Autodesk Inventor part; units mm, degrees
ref_plane "YZ Plane" through (0, 0, 0) normal (1, 0, 0) x (0, 1, 0)
ref_plane "XZ Plane" through (0, 0, 0) normal (0, 1, 0) x (-1, 0, 0)
ref_plane "XY Plane" through (0, 0, 0) normal (0, 0, 1) x (1, 0, 0)
sketch "Sketch1" plane through (0, 0, 0) normal (0, 0, 1) x (1, 0, 0)
  circle A0 centre (0, 0) radius 3
  dimension "Diameter" = 6
extrude "Extrusion1" add sketch "Sketch1" along normal blind 75
sketch "Sketch2" plane through (0, 0, 75) normal (0, 0, 1) x (1, 0, 0)
  circle A0 centre (0, 0) radius 3
  circle A1 centre (0, 0) radius 5
  dimension "Head_Diameter" = 10
extrude "Extrusion2" add sketch "Sketch2" along normal blind 6 contours A0 | A1
sketch "Sketch3" plane through (0, 0, 81) normal (0, 0, 1) x (1, 0, 0)
  circle A0 centre (0, 0) radius 5
  circle A1 centre (0, 0) radius 2.8868 construction
  line L0 (0, 2.8868) -> (2.5, 1.4434)
  line L1 (2.5, -1.4434) -> (2.5, 1.4434)
  line L2 (0, 2.8868) -> (-2.5, 1.4434)
  line L3 (-2.5, -1.4434) -> (-2.5, 1.4434)
  line L4 (-2.5, -1.4434) -> (0, -2.8868)
  line L5 (2.5, -1.4434) -> (0, -2.8868)
  dimension "Hex_Width" = 5
extrude "Extrusion3" cut sketch "Sketch3" against normal blind 3 contours L0 L1 L5 L4 L3 L2
thread "Thread1"
chamfer "Chamfer1" distance 0.6 angle 45 2 edges at (-5, 0, 81) (-3, 0, 0)
equation "\"d9\" = ThreadLength"
equation "\"d12\" = Chamfer"
equation "\"ThreadLength\" = 24"
properties part number "SCREW, SOCKET HD, P, 12.9, M6X1X75MM"
Build history of the part. All positions in model axes, mm. A direction names the side the tool comes from. Round coordinates to 2 decimals unless told otherwise and drop trailing zeros. Loops run counter-clockwise (first coordinate to the right, second up) from the corner with the lowest first, then second, coordinate; pieces in that order, holes last. Notation, with made-up numbers: (32.5, 16) -> (70.5, 16) arc R24 ccw to (70.5, 46) -> close; hole circle Ø3 at (4.25, -19.5). An arc over 180 degrees is marked (long way). One line per item, written item: value. Start each with the question number.
Q1. Cut at B-B on z = 67.5. List the corners of the cut face in (x, y), plus the area to 3 significant figures.
Q2. Cut at A-A on y = 0. List the corners of the cut face in (x, z), plus the area to 3 significant figures.
Q3. Two-plate mould, pull along Y, no slides. Class faces 4 (the face through (-3, 0, 37)), 5 (the face through (-2.5, 0, 80)), 6 (the face through (0, 0, 0)): released by +Y, released by -Y, zero draft, split by the parting line, or undercut.
Q4. Probe line 1 along Z through (x, y) = (-2.5, 3); line 2 along Z through (x, y) = (-1.75, -1.25); line 3 along X through (y, z) = (-4, 77.5). List the from-to ranges inside material, lowest first.
Q5. 3-axis set-ups, long thin cutter, end or side, ignore diameter. For faces 1 (the face through (2, -2, 81)), 2 (the face through (3.3, 0.1, 75)), 3 (the face through (1.233, 2.175, 79.521)): which of +Z, -Z, +X, -X, +Y, -Y reach the whole face in a straight line?
Q6. Drop flat-ended pins along their axis: pin 1 Ø2 at (y, z) = (3, 22.5) entering from +X; pin 2 Ø5 at (y, z) = (-3.5, 15) entering from +X; pin 3 Ø6 at (x, z) = (-2, 22) entering from -Y. Give the stop position or say it passes through.
Computed:
1. outline: circle Ø6 at (0, 0)
1. area: 28.3 mm²
2. outline: (-5, 75) -> (-3, 75) -> (-3, 0.6) -> (-2.4, 0) -> (2.4, 0) -> (3, 0.6) -> (3, 75) -> (5, 75) -> (5, 80.4) -> (4.4, 81) -> (2.5, 81) -> (2.5, 78) -> (-2.5, 78) -> (-2.5, 81) -> (-4.4, 81) -> (-5, 80.4) -> close
2. area: 494 mm²
3. face 4: split by the parting line
3. face 5: undercut
3. face 6: zero draft
4. line 1: 75 to 81
4. line 2: 0 to 78
4. line 3: -3 to 3
5. face 1: +Z, +X, -X, +Y, -Y
5. face 2: -Z
5. face 3: +Z
6. pin 1: x = 2.24
6. pin 2: x = 2.83
6. pin 3: y = -3
